Verification items for this drawing (mm, ordinates from the low corner). A direction names the side the tool comes from. Give positions to 0.01 mm unless a question says otherwise; leave off trailing zeros. Loops run counter-clockwise (first coordinate to the right, second up) from the corner with the lowest first, then second, coordinate; pieces in that order, holes last. Notation, with made-up numbers: M 44.5,81 L 52.5,81 A34 cw 52.5,111 Z; hole C -33.5,-28.75 d1. An arc over 180 degrees is marked long. Write each question's results on one line, items separated by ' | '. Start each with the question number.
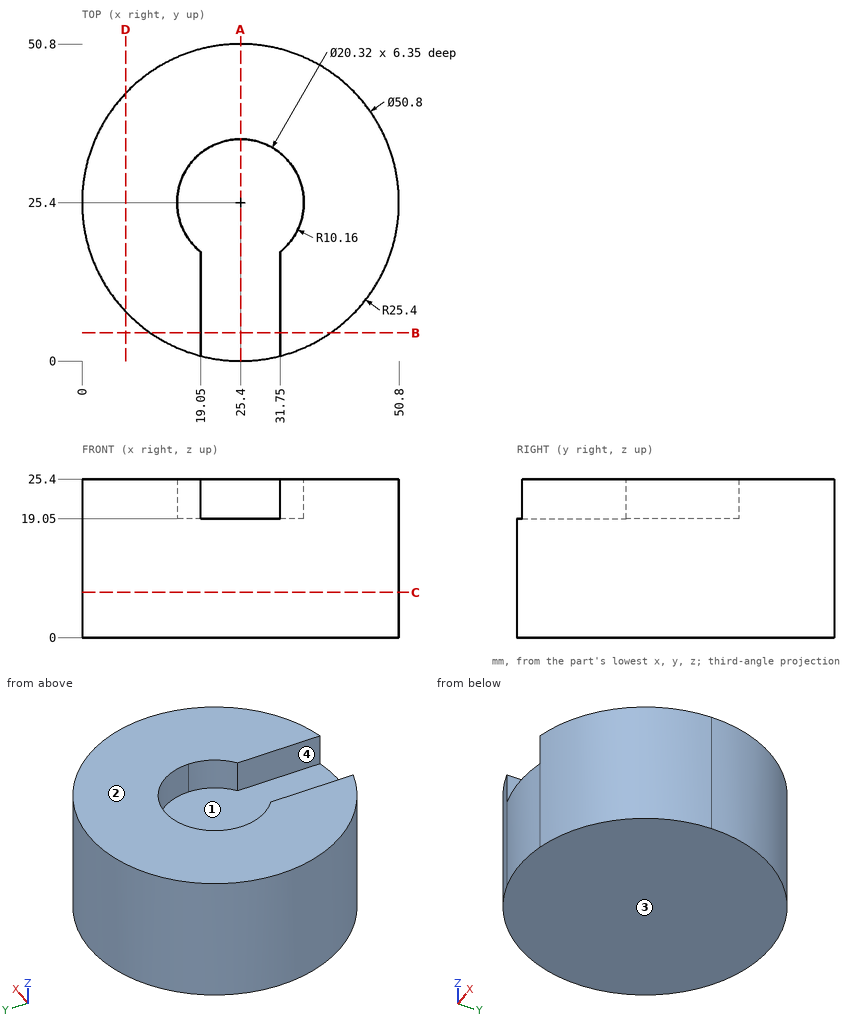
1. Thickness scan on probe 1 along Z at (x, y) = (27, 11); probe 2 along Y at (x, z) = (25.4, 20.75); probe 3 along Y at (x, z) = (25, 12). Record the ranges inside material, lowest first.
2. Depth check by flat-ended pin: pin 1 Ø1.5 at (y, z) = (38, 11) entering from +X; pin 2 Ø3 at (y, z) = (28.5, 20.5) entering from -X; pin 3 Ø1 at (y, z) = (13.5, 12.5) entering from -X. Enter the tip coordinate at first touch or a pass-through.
3. Set-up check for the marked faces 3 and 4: record each of +Z, -Z, +X, -X, +Y, -Y from which the full face is reachable in a straight line by a thin tool's end or side.
4. Section check C-C, the plane z = 7.25. Record the boundary of the cut face in (x, y), plus the area to 3 significant figures.
5. Section check A-A, the plane x = 25.4. Record the boundary of the cut face in (y, z), plus the area to 3 significant figures.
6. Release check for a two-part mould opening along X. For the marked faces 1 and 2 record: released by +X, released by -X, zero draft, split by the parting line, or undercut.
7. Section check B-B, the plane y = 4.5. Record the boundary of the cut face in (x, z).
8. Section check D-D, the plane x = 7. Record the boundary of the cut face in (y, z).
Filled sheet:
1) probe 1: 0 to 19.05 | probe 2: 35.56 to 50.8 | probe 3: 0 to 50.8
2) pin 1: x = 47.87 | pin 2: x = 0.05 | pin 3: x = 2.7
3) face 3: -Z, +X, -X, +Y, -Y | face 4: +Z, -Y
4) outline: M 19.05,0.81 A25.4 ccw 31.75,0.81 A25.4 ccw long Z | area: 2,030 mm2
5) outline: M 0,0 L 50.8,0 L 50.8,25.4 L 35.56,25.4 L 35.56,19.05 L 0,19.05 Z | area: 1,060 mm2
6) face 1: undercut | face 2: zero draft
7) outline: M 10.97,0 L 39.83,0 L 39.83,25.4 L 31.75,25.4 L 31.75,19.05 L 19.05,19.05 L 19.05,25.4 L 10.97,25.4 Z
8) outline: M 7.89,0 L 42.91,0 L 42.91,25.4 L 7.89,25.4 Z
